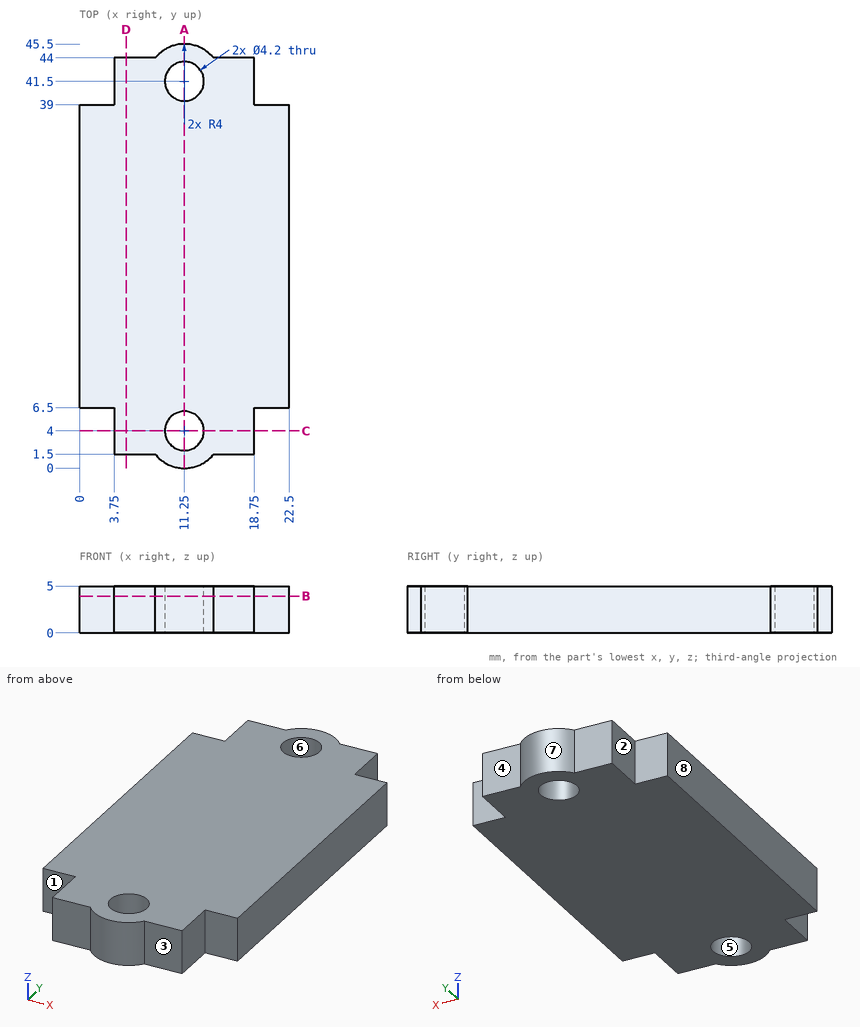
Source: three-view drawing plus pictorial views. Frame: mm from the lowest corner of the part. A direction names the side the tool comes from. Give positions to 0.01 mm unless a question says otherwise; leave off trailing zeros. Write each loop counter-clockwise with the first axis right and the second up, starting at its lowest first coordinate (ties: lowest second). Pieces come first, ordered by that corner, then holes.
(1) Cut plane C-C, the plane y = 4. Return loops of the section in (x, z), then the cut area to 3 significant figures.
(2) Mould query, pull axis X, two halves, no side actions, for the marked faces 6, 7 and 8. Classes: released by +X, released by -X, zero draft, split by the parting line, or undercut.
(3) Access query for the marked faces 1, 2, 3, 4 and 5. Directions: +Z, -Z, +X, -X, +Y, -Y. A direction counts if a zero-diameter tool reaches every point of the face in a straight line with its end or side. Return the directions, or none.
(4) Cut plane D-D, the plane x = 5. Return loops of the section in (y, z), then the cut area to 4 significant figures.
(5) First-contact query: P1, Ø2, axis at x = 6, z = 1.5, coming from the +Y side; P2, Ø1.9, axis at x = 21, z = 3.5, coming from the -Y side; P3, Ø4, axis at x = 15.5, y = 26, coming from the -Z side; P4, Ø2.5, axis at y = 3, z = 3, coming from the +X side. Flat tips, straight axial feed; report the tip coordinate or a pass-through.
(6) Ray query, line 1 (Y direction, x = 11.25, z = 3.2); line 2 (Y direction, x = 4.25, z = 2.2); line 3 (Y direction, x = 20.5, z = 1.5). Return the intervals inside material, ascending.
(7) Cut plane A-A, the plane x = 11.25. Return loops of the section in (y, z).
(8) Cut plane B-B, the plane z = 3.95. Return loops of the section in (x, y), then the cut area to 3 significant figures.
Values follow:
1. outline: (3.75, 0) - (9.15, 0) - (9.15, 5) - (3.75, 5) - close; (13.35, 0) - (18.75, 0) - (18.75, 5) - (13.35, 5) - close
1. area: 54.0 mm2
2. face 6: undercut
2. face 7: split by the parting line
2. face 8: released by -X
3. face 1: +Z, -Z, -X, -Y
3. face 2: +Z, -Z, -X, +Y
3. face 3: +Z, -Z, +X, -Y
3. face 4: +Z, -Z, +X, +Y
3. face 5: +Z, -Z
4. outline: (1.5, 0) - (44, 0) - (44, 5) - (1.5, 5) - close
4. area: 212.5 mm2
5. P1: stops at y = 44
5. P2: stops at y = 6.5
5. P3: stops at z = 0
5. P4: stops at x = 18.75
6. line 1: y = 0 to 1.9, 6.1 to 39.4, 43.6 to 45.5
6. line 2: y = 1.5 to 44
6. line 3: y = 6.5 to 39
7. outline: (0, 0) - (1.9, 0) - (1.9, 5) - (0, 5) - close; (6.1, 0) - (39.4, 0) - (39.4, 5) - (6.1, 5) - close; (43.6, 0) - (45.5, 0) - (45.5, 5) - (43.6, 5) - close
8. outline: (0, 6.5) - (3.75, 6.5) - (3.75, 1.5) - (8.13, 1.5) arc R4 ccw to (14.37, 1.5) - (18.75, 1.5) - (18.75, 6.5) - (22.5, 6.5) - (22.5, 39) - (18.75, 39) - (18.75, 44) - (14.37, 44) arc R4 ccw to (8.13, 44) - (3.75, 44) - (3.75, 39) - (0, 39) - close; hole circle Ø4.2 at (11.25, 4); hole circle Ø4.2 at (11.25, 41.5)
8. area: 867 mm2
